Check sheet for the modelled part. Datum: model origin and axes. Units: mm. A direction names the side the tool comes from. Coordinates: 2 decimals unless noted, no trailing zeros. Loops run counter-clockwise (first coordinate to the right, second up) from the corner with the lowest first, then second, coordinate; pieces in that order, holes last. Notation, with made-up numbers: M 33.5,-34 L 66.5,-34 A26 cw 66.5,-7 Z; hole C 29.5,64 d5. An arc over 180 degrees is marked long. Answer as CSV lines item,"result". Start each with the question number.
from build123d import *

# Parameters (mm, degrees)
SALIENTE_EXTRUIR1_DEPTH = 17
CORTAR_EXTRUIR1_DEPTH   = 8.88
CORTAR_EXTRUIR2_START   = -5.62
CROQUIS6_R              = 99.89
CROQUIS6_R_2            = 93.27
CORTAR_EXTRUIR2_DEPTH   = 3.12
SALIENTE_EXTRUIR3_DEPTH = 17
SALIENTE_EXTRUIR4_START = -5.62
SALIENTE_EXTRUIR4_DEPTH = 11.38
SALIENTE_EXTRUIR5_START = -2.5
SALIENTE_EXTRUIR5_DEPTH = 2.5
REDONDEO1_R             = 50
CROQUIS7_R              = 2.06
SALIENTE_EXTRUIR6_DEPTH = 2.5
REDONDEO7_R             = 5
CROQUIS8_R              = 2.06
CORTAR_EXTRUIR3_DEPTH   = 172.950113436
CROQUIS9_R              = 2.06
CORTAR_EXTRUIR4_DEPTH   = 154.134258449


with BuildPart() as part:
    # Croquis1 → Saliente-Extruir1 (new body)
    with BuildSketch(Plane(origin=(0, 0, 0), x_dir=(0, 0, -1), z_dir=(1, 0, 0))):
        with BuildLine():
            ThreePointArc((70, 74.724240378), (-48.602144929, 90.119607235), (-100.893798125, -17.44))
            Line((-100.893798125, -17.44), (-91.624992769, -17.44))
            ThreePointArc((-91.624992769, -17.44), (-40.990957413, 83.779677192), (70, 61.638404425))
            Line((70, 61.638404425), (70, 74.724240378))
        make_face()
    extrude(amount=SALIENTE_EXTRUIR1_DEPTH)

    # Croquis5 → Cortar-Extruir1 (cut)
    with BuildSketch(Plane.ZY):
        with BuildLine():
            Line((-70, 71.176041615), (-70, 65.359719247))
            ThreePointArc((-70, 65.359719247), (43.12748064, 85.509726427), (94.168674728, -17.44))
            Line((94.168674728, -17.44), (98.294838623, -17.44))
            ThreePointArc((98.294838623, -17.44), (46.5118284, 88.332772621), (-70, 71.176041615))
        make_face()
    extrude(amount=-CORTAR_EXTRUIR1_DEPTH, mode=Mode.SUBTRACT)

    # Croquis6 → Cortar-Extruir2 (cut)
    with BuildSketch(Plane(origin=(17, 0, 0), x_dir=(0, 0, -1), z_dir=(1, 0, 0)).offset(CORTAR_EXTRUIR2_START)):
        Circle(CROQUIS6_R)
        Circle(CROQUIS6_R_2, mode=Mode.SUBTRACT)
    extrude(amount=CORTAR_EXTRUIR2_DEPTH, mode=Mode.SUBTRACT)

    # Croquis2 → Saliente-Extruir3 (add, through all)
    with BuildSketch(Plane(origin=(17, 0, 0), x_dir=(0, 0, -1), z_dir=(1, 0, 0))):
        with BuildLine():
            Line((-111.624992769, -14.94), (-111.624992769, -17.44))
            Line((-111.624992769, -17.44), (-100.893798125, -17.44))
            ThreePointArc((-100.893798125, -17.44), (-101.101710796, -16.19123757), (-101.294168144, -14.94))
            Line((-101.294168144, -14.94), (-111.624992769, -14.94))
        make_face()
    extrude(amount=-SALIENTE_EXTRUIR3_DEPTH)

    # Croquis3 → Saliente-Extruir4 (add)
    with BuildSketch(Plane(origin=(17, 0, 0), x_dir=(0, 0, -1), z_dir=(1, 0, 0)).offset(SALIENTE_EXTRUIR4_START)):
        with BuildLine():
            Line((-91.624992769, -17.44), (-91.624992769, -21.06))
            ThreePointArc((-91.624992769, -21.06), (-92.210779207, -22.474213562), (-93.624992769, -23.06))
            Line((-93.624992769, -23.06), (-109.624992769, -23.06))
            ThreePointArc((-109.624992769, -23.06), (-111.039206332, -22.474213562), (-111.624992769, -21.06))
            Line((-111.624992769, -21.06), (-111.624992769, -20.56))
            Line((-111.624992769, -20.56), (-100.893798125, -20.56))
            Line((-100.893798125, -20.56), (-100.893798125, -17.44))
            Line((-100.893798125, -17.44), (-91.624992769, -17.44))
        make_face()
    extrude(amount=-SALIENTE_EXTRUIR4_DEPTH)

    # Croquis4 → Saliente-Extruir5 (add)
    with BuildSketch(Plane(origin=(17, 0, 0), x_dir=(0, 0, -1), z_dir=(1, 0, 0)).offset(SALIENTE_EXTRUIR5_START)):
        with BuildLine():
            Line((-61.624992769, 70.011807334), (-61.624992769, -17.44))
            Line((-61.624992769, -17.44), (-91.624992769, -17.44))
            ThreePointArc((-91.624992769, -17.44), (-88.223263193, 30.264644911), (-61.624992769, 70.011807334))
        make_face()
    extrude(amount=SALIENTE_EXTRUIR5_DEPTH)

    # Redondeo1
    redondeo1_edges = [part.edges().sort_by_distance(p)[0] for p in [
        (15.75, 70.011807334, 61.624992769),
    ]]
    fillet(redondeo1_edges, radius=REDONDEO1_R)

    # Croquis7 → Saliente-Extruir6 (add)
    with BuildSketch(Plane.XZ.offset(17.44)):
        with BuildLine():
            Line((17, 111.624992769), (27, 111.624992769))
            ThreePointArc((27, 111.624992769), (34.071067812, 108.696060581), (37, 101.624992769))
            Line((37, 101.624992769), (37, 71.624992769))
            ThreePointArc((37, 71.624992769), (34.071067812, 64.553924958), (27, 61.624992769))
            Line((27, 61.624992769), (17, 61.624992769))
            Line((17, 61.624992769), (17, 111.624992769))
        make_face()
        with Locations(Location((27, 101.624992769, 0), (0, 0, 270))):
            Circle(CROQUIS7_R, mode=Mode.SUBTRACT)
        with Locations(Location((27, 71.624992769, 0), (0, 0, 270))):
            Circle(CROQUIS7_R, mode=Mode.SUBTRACT)
    extrude(amount=-SALIENTE_EXTRUIR6_DEPTH)

    # Redondeo7
    redondeo7_edges = [part.edges().sort_by_distance(p)[0] for p in [
        (17, -14.94, 81.459580457),
        (8.5, -14.94, 101.294168144),
    ]]
    fillet(redondeo7_edges, radius=REDONDEO7_R)

    # Croquis8 → Cortar-Extruir3 (cut, through all)
    with BuildSketch(Plane.XZ.offset(23.06)):
        with Locations(Location((5.69, 106.624992769, 0), (0, 0, 171.513837035))):
            Circle(CROQUIS8_R)
    extrude(amount=-CORTAR_EXTRUIR3_DEPTH, mode=Mode.SUBTRACT)

    # Croquis9 → Cortar-Extruir4 (cut, through all)
    with BuildSketch(Plane.ZY.offset(-14.5)):
        with Locations((77.684992769, 6.06)):
            Circle(CROQUIS9_R)
        with Locations((71.624992769, 46.574468299)):
            Circle(CROQUIS9_R)
    extrude(amount=-CORTAR_EXTRUIR4_DEPTH, mode=Mode.SUBTRACT)


solid = part.part
Item 1: Release check for a two-part mould opening along Z. For faces 5 (the face through (4.38, 87.5, 48.06)), 6 (the face through (16, 8, 61.625)), 7 (the face through (17, 55, 60)), 8 (the face through (5.61, 83.02, 42.51)) record: released by +Z, released by -Z, zero draft, split by the parting line, or undercut.
Item 2: Go/stop test with flat-tipped pins: pin 1 (12 mm diameter, centred on x = 9, y = 49.5, fed in from -Z); pin 2 (12 mm diameter, centred on x = 6, z = -36.5, fed in from -Y); pin 3 (1.8 mm diameter, centred on x = 8, y = -18.5, fed in from -Z) (3 decimals). Record where each tip stops, or that it passes through.
Item 3: Material ranges on line 1 (Y direction, x = 8, z = -1) (3 decimals); line 2 (Z direction, x = 6, y = 81); line 3 (Z direction, x = 5.69, y = -21.45) (3 decimals), recorded low to high. Write a range as from..to.
Item 4: Sectioned sample at A-A, the plane y = 81. Record the boundary of the cut face in (x, z), and give its area (3 significant figures).
Item 5: Sectioned sample at C-C, the plane z = 57.5. Record the boundary of the cut face in (x, y), and give its area (3 significant figures).
Item 6: Sectioned sample at B-B, the plane x = 5.69. Record the boundary of the cut face in (y, z) (3 decimals).
Item 7: Sectioned sample at D-D, the plane y = 6.06. Record the boundary of the cut face in (x, z) (3 decimals).
Item 8: Set-up check for faces 1 (the face through (34.148, -16.208, 64.632)), 2 (the face through (27, -14.94, 93)), 3 (the face through (6, -19, 91.625)), 4 (the face through (6, -20.56, 109)): record each of +Z, -Z, +X, -X, +Y, -Y from which the full face is reachable in a straight line by a thin tool's end or side.
Reply:
1,face 5,"undercut"
1,face 6,"released by -Z"
1,face 7,"zero draft"
1,face 8,"undercut"
2,pin 1,"z = 60.57"
2,pin 2,"y = 83.02"
2,pin 3,"z = 91.625"
3,line 1,"93.265..95.765, 99.825..102.385"
3,line 2,"-62.63..-58.35, -51.1..-46.24, 46.24..51.1, 58.35..62.63"
3,line 3,"91.663..104.565, 108.685..111.587"
4,outline,"M 0,-62.63 L 17,-62.63 L 17,-46.24 L 14.5,-46.24 L 14.5,-58.46 L 11.38,-58.46 L 11.38,-46.24 L 0,-46.24 L 0,-51.1 L 8.88,-51.1 L 8.88,-58.35 L 0,-58.35 Z; M 0,46.24 L 11.38,46.24 L 11.38,58.46 L 14.5,58.46 L 14.5,42.51 L 17,42.51 L 17,62.63 L 0,62.63 L 0,58.35 L 8.88,58.35 L 8.88,51.1 L 0,51.1 Z"
4,area,"362 mm²"
5,outline,"M 0,73.44 L 11.38,73.44 L 11.38,81.68 L 14.5,81.68 L 14.5,61.57 L 17,61.57 L 17,84.72 L 0,84.72 L 0,81.61 L 8.88,81.61 L 8.88,76.59 L 0,76.59 Z"
5,area,"151 mm²"
6,outline,"M -23.06,93.625 A2 ccw -21.06,91.625 L -17.44,91.625 A93.27 cw 61.638,-70 L 65.36,-70 A95.77 ccw -17.44,94.169 L -17.44,98.295 A99.83 cw 71.176,-70 L 74.724,-70 A102.39 ccw -9.477,101.95 A5 cw -14.346,104.565 L -17.44,104.565 L -17.44,100.894 L -20.56,100.894 L -20.56,104.565 L -23.06,104.565 Z; M -23.06,108.685 L -20.56,108.685 L -20.56,111.625 L -21.06,111.625 A2 ccw -23.06,109.625 Z; M -17.44,108.685 L -14.94,108.685 L -14.94,111.625 L -17.44,111.625 Z"
7,outline,"M 0,93.073 L 11.38,93.073 L 11.38,99.706 L 14.5,99.706 L 14.5,79.745 L 17,79.745 L 17,102.211 L 0,102.211 L 0,99.646 L 8.88,99.646 L 8.88,95.578 L 0,95.578 Z; M 14.5,61.625 L 17,61.625 L 17,75.625 L 14.5,75.625 Z"
8,face 1,"-Z, +X, +Y, -Y"
8,face 2,"+Z, +X, +Y"
8,face 3,"-Z, +X, -X, -Y"
8,face 4,"+Z, +X, -X"
